Autodesk Inventor part; units mm, degrees
ref_plane "YZ Plane" through (0, 0, 0) normal (1, 0, 0) x (0, 1, 0)
ref_plane "XZ Plane" through (0, 0, 0) normal (0, 1, 0) x (-1, 0, 0)
ref_plane "XY Plane" through (0, 0, 0) normal (0, 0, 1) x (1, 0, 0)
sketch "Sketch2" plane through (0, 0, 0) normal (0, 0, 1) x (1, 0, 0)
  circle A0 centre (-3.175, -1.5465) radius 3.25
  line L0 (-0.0625, 1.7035) -> (7.8834, 1.7035)
  arc A1 (-0.0625, 1.7035) -> (-0.0625, -4.7965) centre (-3.175, -1.5465) ccw
  circle A2 centre (7.8834, -1.5465) radius 3.25
  line L1 (-11.3863, -1.5465) -> (20.6188, -1.5465) construction
  line L2 (-0.0625, -4.7965) -> (7.8834, -4.7965)
  point P0 (9.6395, 1.7844)
  dimension "d6" = 11.0584
  dimension "d7" = 6.5
  dimension "d8" = 6.5
  dimension "d9" = 9
extrude "Extrusion1" add sketch "Sketch2" along normal blind 5 contours A0 | L0 A2 L2 A1 | A2
extrude "Extrusion2" add sketch "Sketch2" against normal blind 5 contours A0
sketch "Sketch3" plane through (0, 0, 5) normal (0, 0, 1) x (1, 0, 0)
  circle A0 centre (7.8834, -1.5465) radius 3.25
  point P0 (0, 0)
extrude "Extrusion3" add sketch "Sketch3" along normal blind 5
equation "\"d7\" = width"
equation "\"d8\" = width"
equation "\"d9\" = R1"
equation "\"d0\" = thickness"
equation "\"d2\" = thickness"
equation "\"d4\" = thickness"
equation "\"R\" = 6.5"
equation "\"thickness\" = 5"
equation "\"width\" = 6.5"
equation "\"R1\" = 9"
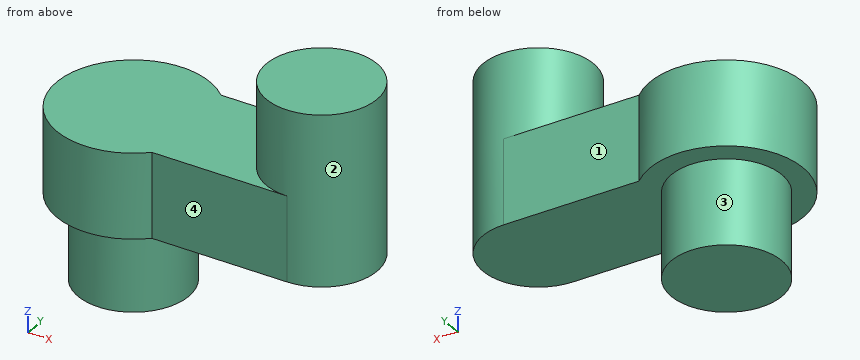
Work out the finished part from the listing and answer in its coordinate system (mm). Face numbers are marked on the shaded views. A direction names the side the tool comes from. Give positions to 0.01 mm unless a question says otherwise; leave off trailing zeros. Loops run counter-clockwise (first coordinate to the right, second up) from the corner with the lowest first, then second, coordinate; pieces in that order, holes last. Notation, with made-up numbers: (81, 85) - (98, 85) arc R27 ccw to (98, 124) - close; hole circle Ø8 at (37, -27.5). An arc over 180 degrees is marked (long way). Answer in a Markdown table with one row per item. Add a question column.
Q1. Each of these flat-tipped pins is pushed along its axis until it touches: P1, Ø3, axis at x = -1, y = -4.5, coming from the +Z side; P2, Ø2.5, axis at x = 4.5, z = 2, coming from the +Y side; P3, Ø1.5, axis at x = 2, z = 2.5, coming from the -Y side. Where does it stop, or does it pass through?
Q2. The part is cut by section D-D (y = -3.75). Determine the outline of the cut face in (x, z), and give its area (3 significant figures).
Q3. Consider line 1 along Z through (x, y) = (8.5, -4); line 2 along Z through (x, y) = (6, -4.25); line 3 along X through (y, z) = (-2, 3). Determine where each line is inside the solid, lowest interval first.
Q4. The part is cut by section B-B (x = -1.75). Determine the outline of the cut face in (y, z), and give its area (3 significant figures).
Q5. A tool of negligible diameter and unlimited length cuts with its end or side. For the marked faces 1, 2, 3 and 4, from which of +Z, -Z, +X, -X, +Y, -Y can it reach the whole face along a straight path? Write none if from no direction.
Q6. The part is cut by section A-A (y = -2.5). Determine the outline of the cut face in (x, z).
Solution:
| question | item | result |
|---|---|---|
| 1 | P1 | stops at z = 5 |
| 1 | P2 | stops at y = 1.7 |
| 1 | P3 | stops at y = -4.8 |
| 2 | outline | (-7.1, 0) - (-5.56, 0) - (-5.56, -5) - (-0.79, -5) - (-0.79, 0) - (10.27, 0) - (10.27, 10) - (5.49, 10) - (5.49, 5) - (-7.1, 5) - close |
| 2 | area | 135 mm² |
| 3 | line 1 | z = 0 to 10 |
| 3 | line 2 | z = 0 to 5 |
| 3 | line 3 | x = -7.65 to 11.1 |
| 4 | outline | (-5.81, 0) - (-4.47, 0) - (-4.47, -5) - (1.37, -5) - (1.37, 0) - (2.72, 0) - (2.72, 5) - (-5.81, 5) - close |
| 4 | area | 71.9 mm² |
| 5 | face 1 | +Z, -Z, +X, +Y |
| 5 | face 2 | +Z |
| 5 | face 3 | -Z |
| 5 | face 4 | +Z, -Z, +X, -Y |
| 6 | outline | (-7.57, 0) - (-6.28, 0) - (-6.28, -5) - (-0.07, -5) - (-0.07, 0) - (10.99, 0) - (10.99, 10) - (4.78, 10) - (4.78, 5) - (-7.57, 5) - close |
